The listing builds one solid part. Answer for the finished solid, in the listing's coordinates (mm). A direction names the side the tool comes from. Round coordinates to 2 decimals unless told otherwise and drop trailing zeros. Order: outer loops, then holes, each group sorted by start corner. A loop starts at its lowest first (then second) coordinate and runs counter-clockwise, first axis right, second up. Notation, with made-up numbers: M -17.75,20.25 L -2.75,20.25 A16 ccw -2.75,29.25 Z; hole C -34.75,50 d1. An arc over 180 degrees is marked long. Write item = value, one per line. Start each with the question number.
(1) A cutting plane is placed at B-B, the plane y = -10.5. Determine the outline of the cut face in (x, z) (3 decimals).
(2) Straight lines are drawn through the part: probe 1 along X at (y, z) = (-18.5, 1.2); probe 2 along Y at (x, z) = (-12, 1.85); probe 3 along X at (y, z) = (-18, 2.3). For each, find the intervals that lie inside material, in ascending order. Write a range as from..to.
(3) Each of these flat-tipped pins is pushed along its axis until it touches: pin 1 (2.5 mm diameter, centred on x = -11.68, y = 2.35, fed in from -Z); pin 2 (1.5 mm diameter, centred on y = 2.5, z = 1, fed in from +X). Where does it stop, or does it pass through?
(4) Which of the six approach directions +Z, -Z, +X, -X, +Y, -Y give full straight-line access (tool end or side, diameter ignored) to faces 1 (the face through (-7.5, 3, 1)), 2 (the face through (-12.89, -25.76, 1.48))?
(5) For a pull along Y with two mould halves and no side action, classify faces 3 (the face through (-13, 5.666, 1)), 4 (the face through (-30, -15, 1)), 5 (the face through (-21.873, -17.603, 1.479)) as released by +Y, released by -Y, zero draft, split by the parting line, or undercut.
(6) A cutting plane is placed at D-D, the plane z = 1.55. Count the separate pieces of the cut face and the enclosed holes in it, and give its area (3 significant figures).
(7) A cutting plane is placed at C-C, the plane y = 3. Determine the outline of the cut face in (x, z).
(8) A cutting plane is placed at A-A, the plane x = -14. Determine the outline of the cut face in (y, z), and give its area (3 significant figures).
from build123d import *

# Parameters (mm, degrees)
EXTRUDE_1_DEPTH      = 3
SKETCH_2_R           = 1.5
CUT_EXTRUDE_7_DEPTH  = 43.02014847
SKETCH_4_R           = 1.5
CUT_EXTRUDE_8_DEPTH  = 43.02014847
SKETCH_6_R           = 10.5
SKETCH_6_R_2         = 3.01
CUT_EXTRUDE_9_DEPTH  = 43.02014847
SKETCH_7_R           = 1.5
CUT_EXTRUDE_10_DEPTH = 43.02014847


with BuildPart() as part:
    # 草图1 → 凸台-拉伸1 (new body)
    with BuildSketch(Plane.XY):
        Polygon((-7.5, 0), (7.5, 0), (7.5, 5.665837688), (17.5, 5.665837688), (30, -1.269316313), (30, -29.269316313), (-30, -29.269316313), (-30, -1.269316313), (-17.5, 5.665837688), (-7.5, 5.665837688), align=None)
    extrude(amount=EXTRUDE_1_DEPTH)

    # 草图2 → 切除-拉伸7 (cut, through all)
    with BuildSketch(Plane(origin=(0, 0, 0), x_dir=(-1, 0, 0), z_dir=(0, 0, -1))):
        with Locations((-25.62844718, -17.669380188)):
            Circle(SKETCH_2_R)
        with Locations((-25.62844718, -7.669380188)):
            Circle(SKETCH_2_R)
        with Locations((23.37155282, -17.669380188)):
            Circle(SKETCH_2_R)
        with Locations((23.37155282, -7.669380188)):
            Circle(SKETCH_2_R)
    extrude(amount=-CUT_EXTRUDE_7_DEPTH, mode=Mode.SUBTRACT)

    # 草图4 → 切除-拉伸8 (cut, through all)
    with BuildSketch(Plane(origin=(0, 0, 0), x_dir=(-1, 0, 0), z_dir=(0, 0, -1))):
        with Locations((-11.696832964, 2.350343297)):
            Circle(SKETCH_4_R)
        with Locations((11.682164636, 2.350343297)):
            Circle(SKETCH_4_R)
    extrude(amount=-CUT_EXTRUDE_8_DEPTH, mode=Mode.SUBTRACT)

    # 草图6 → 切除-拉伸9 (cut, through all)
    with BuildSketch(Plane(origin=(0, 0, 0), x_dir=(-1, 0, 0), z_dir=(0, 0, -1))):
        with Locations((-12.15844718, -12.669380188)):
            Circle(SKETCH_6_R)
        with Locations((10.34155282, -12.669316313)):
            Circle(SKETCH_6_R_2)
    extrude(amount=-CUT_EXTRUDE_9_DEPTH, mode=Mode.SUBTRACT)

    # 草图7 → 切除-拉伸10 (cut, through all)
    with BuildSketch(Plane(origin=(0, 0, 0), x_dir=(-1, 0, 0), z_dir=(0, 0, -1))):
        with Locations((14, -26.769316313)):
            Circle(SKETCH_7_R)
        with Locations((-14, -26.769316313)):
            Circle(SKETCH_7_R)
    extrude(amount=-CUT_EXTRUDE_10_DEPTH, mode=Mode.SUBTRACT)


solid = part.part
Reported:
q1.outline = M -30,0 L -12.428,0 L -12.428,3 L -30,3 Z; M -8.255,0 L 1.885,0 L 1.885,3 L -8.255,3 Z; M 22.432,0 L 30,0 L 30,3 L 22.432,3 Z
q2.probe_1 = -30..-24.62, -22.12..3.43, 20.89..24.38, 26.88..30
q2.probe_2 = -29.27..-15.18, -10.16..0.88, 3.82..5.67
q2.probe_3 = -30..-24.83, -21.91..3.11, 21.2..24.17, 27.09..30
q3.pin_1 = through
q3.pin_2 = 24.56
q4.face_1 = +Z, -Z, +Y
q4.face_2 = +Z, -Z
q5.face_3 = released by +Y
q5.face_4 = zero draft
q5.face_5 = undercut
q6.separate_pieces = 1
q6.enclosed_holes = 10
q6.area = 1,490 mm²
q7.outline = M -22.3,0 L -13.03,0 L -13.03,3 L -22.3,3 Z; M -10.33,0 L -7.5,0 L -7.5,3 L -10.33,3 Z; M 7.5,0 L 10.34,0 L 10.34,3 L 7.5,3 Z; M 13.05,0 L 22.3,0 L 22.3,3 L 13.05,3 Z
q8.outline = M -29.27,0 L -28.27,0 L -28.27,3 L -29.27,3 Z; M -25.27,0 L 5.67,0 L 5.67,3 L -25.27,3 Z
q8.area = 95.8 mm²
